from build123d import *

# Parameters (mm, degrees)
ESQUISSE1_W             = 60
ESQUISSE1_H             = 40
BOSS_EXTRU_1_DEPTH      = 2
ESQUISSE2_W             = 55
ESQUISSE2_H             = 35
BOSS_EXTRU_2_DEPTH      = 10
CONG_1_R                = 3
CONG_2_R                = 1
ESQUISSE3_W             = 47
ESQUISSE3_H             = 27
ENL_V_MAT_EXTRU_1_DEPTH = 10
ESQUISSE4_R             = 1.5
ENL_V_MAT_EXTRU_2_DEPTH = 72.765242283


with BuildPart() as part:
    # Esquisse1 → Boss.-Extru.1 (new body)
    with BuildSketch(Plane.XY):
        with Locations((30, 20)):
            Rectangle(ESQUISSE1_W, ESQUISSE1_H)
    extrude(amount=BOSS_EXTRU_1_DEPTH)

    # Esquisse2 → Boss.-Extru.2 (add)
    with BuildSketch(Plane.XY.offset(2)):
        with Locations((30, 20)):
            Rectangle(ESQUISSE2_W, ESQUISSE2_H)
    extrude(amount=BOSS_EXTRU_2_DEPTH)

    # Congé1
    cong_1_edges = [part.edges().sort_by_distance(p)[0] for p in [
        (57.5, 37.5, 7),
        (2.5, 37.5, 7),
        (2.5, 2.5, 7),
        (57.5, 2.5, 7),
    ]]
    fillet(cong_1_edges, radius=CONG_1_R)

    # Congé2
    cong_2_edges = [part.edges().sort_by_distance(p)[0] for p in [
        (0, 40, 1),
        (60, 40, 1),
        (60, 0, 1),
        (0, 0, 1),
    ]]
    fillet(cong_2_edges, radius=CONG_2_R)

    # Esquisse3 → Enlèv. mat.-Extru.1 (cut)
    with BuildSketch(Plane.XY.offset(12)):
        with Locations((30, 20)):
            Rectangle(ESQUISSE3_W, ESQUISSE3_H)
    extrude(amount=-ENL_V_MAT_EXTRU_1_DEPTH, mode=Mode.SUBTRACT)

    # Esquisse4 → Enlèv. mat.-Extru.2 (cut, through all)
    with BuildSketch(Plane(origin=(0, 37.5, 0), x_dir=(1, 0, 0), z_dir=(0, 1, 0))):
        with Locations(Location((30, -7, 0), (0, 0, 270))):
            Circle(ESQUISSE4_R)
    extrude(amount=-ENL_V_MAT_EXTRU_2_DEPTH, mode=Mode.SUBTRACT)


solid = part.part
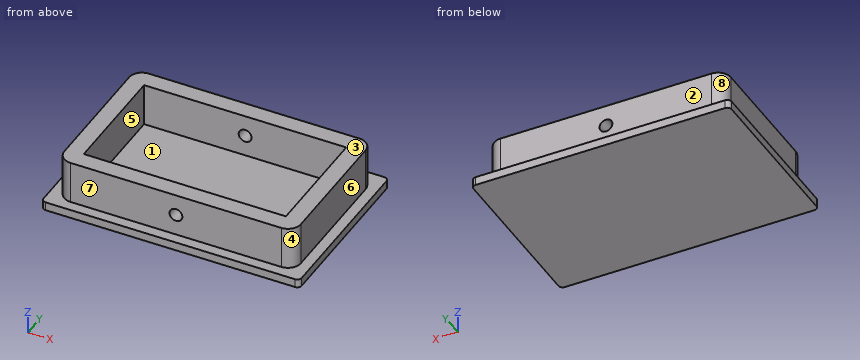
Work out the finished part from the listing and answer in its coordinate system (mm). Face numbers are marked on the shaded views. A direction names the side the tool comes from. Give positions to 0.01 mm unless a question says otherwise; leave off trailing zeros. Order: outer loops, then holes, each group sorted by start corner. A loop starts at its lowest first (then second) coordinate and runs counter-clockwise, first axis right, second up. Notation, with made-up numbers: (56.5, 7) -> (79.5, 7) arc R21 cw to (79.5, 36) -> close; hole circle Ø7 at (-5.5, 81). An arc over 180 degrees is marked (long way). Answer as a JSON object with one key per item and string values. Group by question number.
1. Section B-B on x = 30 is taken. Determine the outline of the cut face in (y, z), plus the area to 3 significant figures.
2. A tool of negligible diameter and unlimited length cuts with its end or side. For the marked faces 1, 2, 3 and 4, from which of +Z, -Z, +X, -X, +Y, -Y can it reach the whole face along a straight path? Write none if from no direction.
3. Section D-D on y = 22 is taken. Determine the outline of the cut face in (x, z), plus the area to 3 significant figures.
4. Flat-ended cylindrical pins translate along their axes: pin 1 Ø3 at (y, z) = (22.5, 5.5) entering from -X; pin 2 Ø21.5 at (x, y) = (36.5, 18) entering from +Z; pin 3 Ø5 at (x, z) = (20, 8.5) entering from -Y; pin 4 Ø4 at (x, y) = (46.5, 18.5) entering from -Z. Find the tip coordinate at first contact, or state that the pin passes through.
5. The mould has two halves that part along X. Classify the marked faces 5, 6, 7 and 8: released by +X, released by -X, zero draft, split by the parting line, or undercut.
6. Section C-C on z = 4 is taken. Determine the outline of the cut face in (x, y), plus the area to 3 significant figures.
7. Consider line 1 along Y through (x, z) = (45.5, 10.5); line 2 along X through (y, z) = (34.35, 7); line 3 along X through (y, z) = (25.5, 10). Determine where each line is inside the solid, lowest interval first. Write a range as [from, to].
8. Section A-A on z = 7 is taken. Determine the outline of the cut face in (x, y), plus the area to 3 significant figures.
Result sheet:
{
 "1": {"outline": "(0, 0) -> (40, 0) -> (40, 2) -> (37.5, 2) -> (37.5, 5.5) -> (33.5, 5.5) -> (33.5, 2) -> (6.5, 2) -> (6.5, 5.5) -> (2.5, 5.5) -> (2.5, 2) -> (0, 2) -> close; (2.5, 8.5) -> (6.5, 8.5) -> (6.5, 12) -> (2.5, 12) -> close; (33.5, 8.5) -> (37.5, 8.5) -> (37.5, 12) -> (33.5, 12) -> close", "area": "136 mm^2"},
 "2": {"face 1": "+Z", "face 2": "+Z, +X, -X, +Y", "face 3": "+Z, +X, -X, +Y, -Y", "face 4": "+Z, +X, -Y"},
 "3": {"outline": "(0, 0) -> (60, 0) -> (60, 2) -> (57.5, 2) -> (57.5, 12) -> (53.5, 12) -> (53.5, 2) -> (6.5, 2) -> (6.5, 12) -> (2.5, 12) -> (2.5, 2) -> (0, 2) -> close", "area": "200 mm^2"},
 "4": {"pin 1": "stops at x = 2.5", "pin 2": "stops at z = 2", "pin 3": "stops at y = 2.5", "pin 4": "stops at z = 0"},
 "5": {"face 5": "undercut", "face 6": "released by +X", "face 7": "zero draft", "face 8": "released by -X"},
 "6": {"outline": "(2.5, 5.5) arc R3 ccw to (5.5, 2.5) -> (54.5, 2.5) arc R3 ccw to (57.5, 5.5) -> (57.5, 34.5) arc R3 ccw to (54.5, 37.5) -> (5.5, 37.5) arc R3 ccw to (2.5, 34.5) -> close; hole (6.5, 6.5) -> (53.5, 6.5) -> (53.5, 33.5) -> (6.5, 33.5) -> close", "area": "648 mm^2"},
 "7": {"line 1": "y = [2.5, 6.5], [33.5, 37.5]", "line 2": "x = [2.5, 28.5], [31.5, 57.5]", "line 3": "x = [2.5, 6.5], [53.5, 57.5]"},
 "8": {"outline": "(2.5, 5.5) arc R3 ccw to (5.5, 2.5) -> (28.5, 2.5) -> (28.5, 6.5) -> (6.5, 6.5) -> (6.5, 33.5) -> (28.5, 33.5) -> (28.5, 37.5) -> (5.5, 37.5) arc R3 ccw to (2.5, 34.5) -> close; (31.5, 2.5) -> (54.5, 2.5) arc R3 ccw to (57.5, 5.5) -> (57.5, 34.5) arc R3 ccw to (54.5, 37.5) -> (31.5, 37.5) -> (31.5, 33.5) -> (53.5, 33.5) -> (53.5, 6.5) -> (31.5, 6.5) -> close", "area": "624 mm^2"}
}
